Could you check a few things on this model? Use its own coordinates, in mm. A direction names the side the tool comes from. Give positions to 0.01 mm unless a question says otherwise; leave off trailing zeros. Order: outer loops, then holes, each group sorted by start corner. A loop starts at its lowest first (then second) coordinate and runs counter-clockwise, first axis right, second up. Notation, with made-up numbers: (-11, -5) -> (9, -5) arc R19 ccw to (9, 32) -> close; hole circle Ø6 at (-33.5, 47). An arc over 180 degrees is marked (long way). Use one line per item in the form item = value. Start each with the question number.
from build123d import *

# Parameters (mm, degrees)
BOSS_EXTRUDE1_DEPTH = 8
SHELL1_T            = -1.6


with BuildPart() as part:
    # Sketch1 → Boss-Extrude1 (new body)
    with BuildSketch(Plane.XY):
        Polygon((-8, 9.6), (8, 9.6), (16, 0), (-16, 0), align=None)
    extrude(amount=BOSS_EXTRUDE1_DEPTH)

    # Sketch2 → section 1 of loft1
    with BuildSketch(Plane.XY.offset(32), mode=Mode.PRIVATE) as loft1_s1:
        with BuildLine():
            Line((-8, 0), (8, 0))
            Line((8, 0), (6.75, 1.5))
            Line((6.75, 1.5), (-6.75, 1.5))
            Line((-6.75, 1.5), (-8, 0))
        make_face()
    # loft from a face of the part (loft1)
    loft([part.faces().sort_by_distance((0, 4.266666667, 8))[0], loft1_s1.sketch])

    # Shell1
    shell1_openings = [part.faces().sort_by_distance(p)[0] for p in [
        (0, 0, 14.153846154),
    ]]
    offset(amount=SHELL1_T, openings=shell1_openings)


solid = part.part
(1) I'm going to push flat-ended pins straight in: pin 1 Ø12 at (x, z) = (4, 28) entering from +Y (3 decimals); pin 2 Ø3 at (x, z) = (-12, 9) entering from +Y; pin 3 Ø1.8 at (x, z) = (-2.5, 4.5) entering from -Y. Where does each tip first touch, or does it pass through?
(2) Please list where these lines run through material, in increasing order: probe 1 along X at (y, z) = (1.75, 19) (3 decimals); probe 2 along X at (y, z) = (4.5, 5); probe 3 along Y at (x, z) = (-2, 3.5).
(3) Imagine slicing it at A-A (z = 4). Write out the boundary of the cut face in (x, y), plus the area to 3 significant figures.
(4) We'd pull the mould along Z, two halves only. Please class faces 1 (the flat face through (-12.06, 4.73, 3.94)), 2 (the flat face through (0, 4, 0)), 3 (the flat face through (-10.631, 3.944, 4.656)): pulls with the +Z half, pulls with the -Z half, needs draft (parallel to the pull), parting line crosses it, or undercut.
(5) Which directions (+Z, -Z, +X, -X, +Y, -Y) give clear straight access to the entire face, cutting with the end or side of a thin tool? Please do faces 4 (the flat face through (10.5, 4.1, 4.7)), 5 (the flat face through (0, 1, 32)).
Calculated:
q1.pin_1 = 4.875
q1.pin_2 = 6.3
q1.pin_3 = 8
q2.probe_1 = -10.875 to -8.725, 8.725 to 10.875
q2.probe_2 = -12.25 to -10.17, 10.17 to 12.25
q2.probe_3 = 8 to 9.6
q3.outline = (-16, 0) -> (-13.92, 0) -> (-7.25, 8) -> (7.25, 8) -> (13.92, 0) -> (16, 0) -> (8, 9.6) -> (-8, 9.6) -> close
q3.area = 61.1 mm2
q4.face_1 = needs draft
q4.face_2 = pulls with the -Z half
q4.face_3 = undercut
q5.face_4 = -Y
q5.face_5 = +Z, +X, -X, +Y, -Y
